Model file for the job. Use its own axes, mm. Face numbers are marked on the shaded views. A direction names the side the tool comes from. Coordinates: 2 decimals unless noted, no trailing zeros. Write each loop counter-clockwise with the first axis right and the second up, starting at its lowest first coordinate (ties: lowest second). Pieces come first, ordered by that corner, then holes. Notation, with made-up numbers: (-13, -1) -> (31, -1) arc R16 ccw to (31, 21) -> close; hole circle Ø6 at (80.5, -32). An arc over 180 degrees is marked (long way). Answer as a JSON object with one key per item and string values. Group by question number.
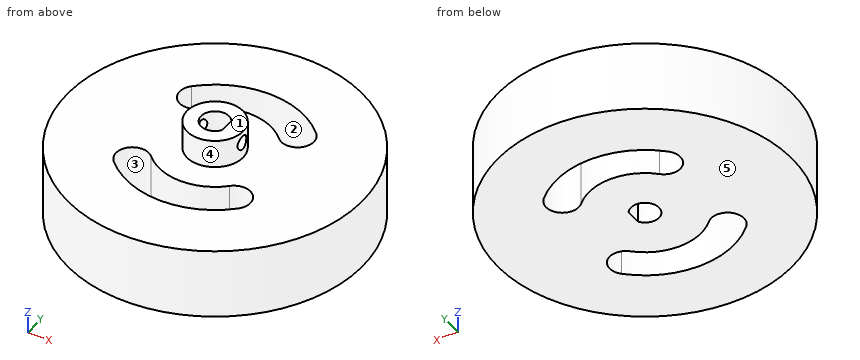
from build123d import *

# Parameters (mm, degrees)
SKETCH_1_R               = 31.5
EXTRUDE_1_DEPTH          = 15
SKETCH_3_R               = 3
CUT_EXTRUDE_2_DEPTH      = 48.005318848
SKETCH_14_R              = 6
SKETCH_14_R_2            = 3
EXTRUDE_3_DEPTH          = 6
EXTRUDE_START            = -21
EXTRUDE_4_DEPTH          = 21
CUT_EXTRUDE_3_DEPTH      = 50.249365478
CUT_EXTRUDE_3_DEPTH_BACK = 50.249365478
SKETCH_18_R              = 1.5
CUT_EXTRUDE_5_DEPTH      = 48.00531888
CUT_EXTRUDE_5_DEPTH_BACK = 48.00531888


with BuildPart() as part:
    # 草图1 → 凸台-拉伸1 (new body)
    with BuildSketch(Plane.XY):
        Circle(SKETCH_1_R)
    extrude(amount=EXTRUDE_1_DEPTH)

    # 草图3 → 切除-拉伸2 (cut, through all)
    with BuildSketch(Plane(origin=(0, 0, 0), x_dir=(-1, 0, 0), z_dir=(0, 0, -1))):
        Circle(SKETCH_3_R)
    extrude(amount=-CUT_EXTRUDE_2_DEPTH, mode=Mode.SUBTRACT)

    # 草图14 → 凸台-拉伸3 (add)
    with BuildSketch(Plane.XY.offset(15)):
        Circle(SKETCH_14_R)
        with Locations(Location((0, 0, 0), (0, 0, 180))):
            Circle(SKETCH_14_R_2, mode=Mode.SUBTRACT)
    extrude(amount=EXTRUDE_3_DEPTH)

    # 草图19 → 凸台-拉伸4 (add)
    with BuildSketch(Plane.XY.offset(21).offset(EXTRUDE_START)):
        with BuildLine():
            Line((2.5, 1.658312395), (2.5, -1.658312395))
            ThreePointArc((2.5, -1.658312395), (3, 0), (2.5, 1.658312395))
        make_face()
    extrude(amount=EXTRUDE_4_DEPTH)

    # 草图18 → 切除-拉伸3 (cut, two sides: drawn at the far end of the back side and taken through both)
    with BuildSketch(Plane(origin=(0, 0, 0), x_dir=(0, 0, -1), z_dir=(1, 0, 0)).offset(-CUT_EXTRUDE_3_DEPTH_BACK)):
        with Locations(Location((-18.5, 0, 0), (0, 0, 180))):
            Circle(SKETCH_18_R)
    extrude(amount=CUT_EXTRUDE_3_DEPTH + CUT_EXTRUDE_3_DEPTH_BACK, mode=Mode.SUBTRACT)

    # 草图20 → 切除-拉伸5 (cut, two sides: drawn at the far end of the back side and taken through both)
    with BuildSketch(Plane.XY.offset(15).offset(-CUT_EXTRUDE_5_DEPTH_BACK)):
        with BuildLine():
            ThreePointArc((8.485281374, 8.485281374), (0, 12), (-8.485281374, 8.485281374))
            ThreePointArc((-8.485281374, 8.485281374), (-13.435028843, 8.485281374), (-13.435028843, 13.435028843))
            ThreePointArc((-13.435028843, 13.435028843), (0, 19), (13.435028843, 13.435028843))
            ThreePointArc((13.435028843, 13.435028843), (13.435028843, 8.485281374), (8.485281374, 8.485281374))
        make_face()
        with BuildLine():
            ThreePointArc((8.485281374, -8.485281374), (13.435028843, -8.485281374), (13.435028843, -13.435028843))
            ThreePointArc((13.435028843, -13.435028843), (0, -19), (-13.435028843, -13.435028843))
            ThreePointArc((-13.435028843, -13.435028843), (-13.435028843, -8.485281374), (-8.485281374, -8.485281374))
            ThreePointArc((-8.485281374, -8.485281374), (0, -12), (8.485281374, -8.485281374))
        make_face()
    extrude(amount=CUT_EXTRUDE_5_DEPTH + CUT_EXTRUDE_5_DEPTH_BACK, mode=Mode.SUBTRACT)


solid = part.part
(1) Cut at C-C on z = 18.5. List the corners of the cut face in (x, y).
(2) Cut at A-A on x = 0. List the corners of the cut face in (y, z), plus the area to 3 significant figures.
(3) Wall check: probe 1 along Y at (x, z) = (0, 7); probe 2 along Y at (x, z) = (-7.5, 6.5); probe 3 along Z at (x, y) = (22, 16). Give the ranges that are in metal, low to high.
(4) Cut at D-D on y = 18. List the corners of the cut face in (x, z), plus the area to 3 significant figures.
(5) Cut at B-B on y = 0. List the corners of the cut face in (x, z), plus the area to 3 significant figures.
(6) Pin check, flat tips, straight feed: pin 1 (8 mm diameter, centred on y = 6, z = 16.5, fed in from +X); pin 2 (4 mm diameter, centred on x = 16, y = 11, fed in from +Z); pin 3 (1.7 mm diameter, centred on y = 1, z = 14.5, fed in from -X); pin 4 (1.8 mm diameter, centred on y = 0, z = 18.5, fed in from +X). Stop position of each tip, or through.
(7) 3-axis set-ups, long thin cutter, end or side, ignore diameter. For the marked faces 1 and 2: which of +Z, -Z, +X, -X, +Y, -Y reach the whole face in a straight line?
(8) Pull direction Y, two halves, no side cores. Call the marked faces 3, 4 and 5: released by +Y, released by -Y, zero draft, split by the parting line, or undercut.
Results found:
{
 "1": {"outline": "(-5.81, -1.5) arc R6 ccw to (5.81, -1.5) -> (2.5, -1.5) -> (2.5, -1.66) arc R3 cw to (-2.6, -1.5) -> close; (-5.81, 1.5) -> (-2.6, 1.5) arc R3 cw to (2.5, 1.66) -> (2.5, 1.5) -> (5.81, 1.5) arc R6 ccw to start"},
 "2": {"outline": "(-31.5, 0) -> (-19, 0) -> (-19, 15) -> (-31.5, 15) -> close; (-12, 0) -> (-3, 0) -> (-3, 21) -> (-6, 21) -> (-6, 15) -> (-12, 15) -> close; (3, 0) -> (12, 0) -> (12, 15) -> (6, 15) -> (6, 21) -> (3, 21) -> close; (19, 0) -> (31.5, 0) -> (31.5, 15) -> (19, 15) -> close", "area": "681 mm²"},
 "3": {"probe 1": "y = -31.5 to -19, -12 to -3, 3 to 12, 19 to 31.5", "probe 2": "y = -30.59 to -17.46, -9.37 to 9.37, 17.46 to 30.59", "probe 3": "z = 0 to 15"},
 "4": {"outline": "(-25.85, 0) -> (-6.08, 0) -> (-6.08, 15) -> (-25.85, 15) -> close; (6.08, 0) -> (25.85, 0) -> (25.85, 15) -> (6.08, 15) -> close", "area": "593 mm²"},
 "5": {"outline": "(-31.5, 0) -> (-3, 0) -> (-3, 17) -> (-6, 17) -> (-6, 15) -> (-31.5, 15) -> close; (-6, 20) -> (-3, 20) -> (-3, 21) -> (-6, 21) -> close; (2.5, 0) -> (31.5, 0) -> (31.5, 15) -> (6, 15) -> (6, 17) -> (2.5, 17) -> close; (2.5, 20) -> (6, 20) -> (6, 21) -> (2.5, 21) -> close", "area": "882 mm²"},
 "6": {"pin 1": "stops at x = 31.42", "pin 2": "stops at z = 15", "pin 3": "stops at x = -31.5", "pin 4": "passes through"},
 "7": {"face 1": "+Z, +X, -X, +Y, -Y", "face 2": "+Z, -Z"},
 "8": {"face 3": "undercut", "face 4": "split by the parting line", "face 5": "zero draft"}
}
